from build123d import *

# Parameters (mm, degrees)
SKETCH_1_W          = 13.5
SKETCH_1_H          = 25
SKETCH_1_W_2        = 2.5
SKETCH_1_H_2        = 4.75
EXTRUDE_1_DEPTH     = 1.2
SKETCH_2_R          = 1.7
CUT_EXTRUDE_1_DEPTH = 1.2
SKETCH_3_R          = 2.1
EXTRUDE_2_DEPTH     = 25
SKETCH_4_R          = 1.5
CUT_EXTRUDE_2_DEPTH = 25
SKETCH_5_W          = 5
SKETCH_5_H          = 15.5
CUT_EXTRUDE_3_DEPTH = 7.5


with BuildPart() as part:
    # 草图1 → 凸台-拉伸1 (new body)
    with BuildSketch(Plane.XY):
        with Locations((6.75, 0)):
            Rectangle(SKETCH_1_W, SKETCH_1_H)
        with Locations((-1.25, 10.125)):
            Rectangle(SKETCH_1_W_2, SKETCH_1_H_2)
        with Locations((-1.25, -10.125)):
            Rectangle(SKETCH_1_W_2, SKETCH_1_H_2)
    extrude(amount=EXTRUDE_1_DEPTH)

    # 草图2 → 切除-拉伸1 (cut)
    with BuildSketch(Plane.XY.offset(1.2)):
        with Locations((8.5, 7)):
            Circle(SKETCH_2_R)
        with Locations((8.5, -7)):
            Circle(SKETCH_2_R)
    extrude(amount=-CUT_EXTRUDE_1_DEPTH, mode=Mode.SUBTRACT)

    # 草图3 → 凸台-拉伸2 (add)
    with BuildSketch(Plane.XZ.offset(12.5)):
        with Locations(Location((-2.5, 2.1, 0), (0, 0, 270))):
            Circle(SKETCH_3_R)
    extrude(amount=-EXTRUDE_2_DEPTH)

    # 草图4 → 切除-拉伸2 (cut)
    with BuildSketch(Plane.XZ.offset(12.5)):
        with Locations(Location((-2.5, 2.1, 0), (0, 0, 270))):
            Circle(SKETCH_4_R)
    extrude(amount=-CUT_EXTRUDE_2_DEPTH, mode=Mode.SUBTRACT)

    # 草图5 → 切除-拉伸3 (cut, symmetric)
    with BuildSketch(Plane.XY.offset(1.2)):
        with Locations((-2.5, 0)):
            Rectangle(SKETCH_5_W, SKETCH_5_H)
    extrude(amount=CUT_EXTRUDE_3_DEPTH, both=True, mode=Mode.SUBTRACT)


solid = part.part
Model file for the job. Use its own axes, mm. A direction names the side the tool comes from. Give positions to 0.01 mm unless a question says otherwise; leave off trailing zeros. Loops run counter-clockwise (first coordinate to the right, second up) from the corner with the lowest first, then second, coordinate; pieces in that order, holes last. Notation, with made-up numbers: (-28.75, 53) - (-5.75, 53) arc R20 ccw to (-5.75, 81) - close; hole circle Ø2 at (-12, -29.75). An arc over 180 degrees is marked (long way). Use one line per item in the form item = value.
(1) Drop flat-ended pins along their axis: P1, Ø3, axis at x = 3.5, y = 9.5, coming from the +Z side; P2, Ø3, axis at x = 8.5, y = 7, coming from the +Z side. Give the stop position or say it passes through.
Determined:
P1 = 1.2
P2 = through
(2) Cut at A-A (y = -7). Give the cut face in (x, z), then the cut area to 3 significant figures.
Determined:
outline = (0, 0) - (6.8, 0) - (6.8, 1.2) - (0, 1.2) - close; (10.2, 0) - (13.5, 0) - (13.5, 1.2) - (10.2, 1.2) - close
area = 12.1 mm^2
(3) Cut at C-C (z = 2.1). Give the cut face in (x, y).
Determined:
outline = (-4.6, -12.5) - (-4, -12.5) - (-4, -7.75) - (-4.6, -7.75) - close; (-4.6, 7.75) - (-4, 7.75) - (-4, 12.5) - (-4.6, 12.5) - close; (-1, -12.5) - (-0.4, -12.5) - (-0.4, -7.75) - (-1, -7.75) - close; (-1, 7.75) - (-0.4, 7.75) - (-0.4, 12.5) - (-1, 12.5) - close
(4) Pull direction X, two halves, no side cores. Call faces 3 (the face through (-1, 7.75, 1)), 4 (the face through (13.5, 0, 1)), 5 (the face through (8.13, -8.66, 0.61)): pulls with the +X half, pulls with the -X half, needs draft (parallel to the pull), parting line crosses it, or undercut.
Determined:
face_3 = needs draft
face_4 = pulls with the +X half
face_5 = undercut
(5) Cut at B-B (x = 8.5). Give the cut face in (y, z), then the cut area to 3 significant figures.
Determined:
outline = (-12.5, 0) - (-8.7, 0) - (-8.7, 1.2) - (-12.5, 1.2) - close; (-5.3, 0) - (5.3, 0) - (5.3, 1.2) - (-5.3, 1.2) - close; (8.7, 0) - (12.5, 0) - (12.5, 1.2) - (8.7, 1.2) - close
area = 21.8 mm^2
(6) Cut at D-D (x = -2). Give the cut face in (y, z).
Determined:
outline = (-12.5, 0) - (-7.75, 0) - (-7.75, 0.69) - (-12.5, 0.69) - close; (-12.5, 3.51) - (-7.75, 3.51) - (-7.75, 4.14) - (-12.5, 4.14) - close; (7.75, 0) - (12.5, 0) - (12.5, 0.69) - (7.75, 0.69) - close; (7.75, 3.51) - (12.5, 3.51) - (12.5, 4.14) - (7.75, 4.14) - close
(7) Drill centre lines: L1, parallel to Y at x = 8.5, z = 0.55; L2, parallel to Y at x = -0.25, z = 0.3; L3, parallel to X at y = -8.85, z = 2.1. Where is each one in solid material? Low to high.
Determined:
L1 = -12.5 to -8.7, -5.3 to 5.3, 8.7 to 12.5
L2 = -12.5 to -7.75, 7.75 to 12.5
L3 = -4.6 to -4, -1 to -0.4
(8) 3-axis set-ups, long thin cutter, end or side, ignore diameter. For faces 1 (the face through (0, 0, 1)), 2 (the face through (8.13, 5.34, 0.61)): which of +Z, -Z, +X, -X, +Y, -Y reach the whole face in a straight line?
Determined:
face_1 = +Z, -Z, -X
face_2 = +Z, -Z
